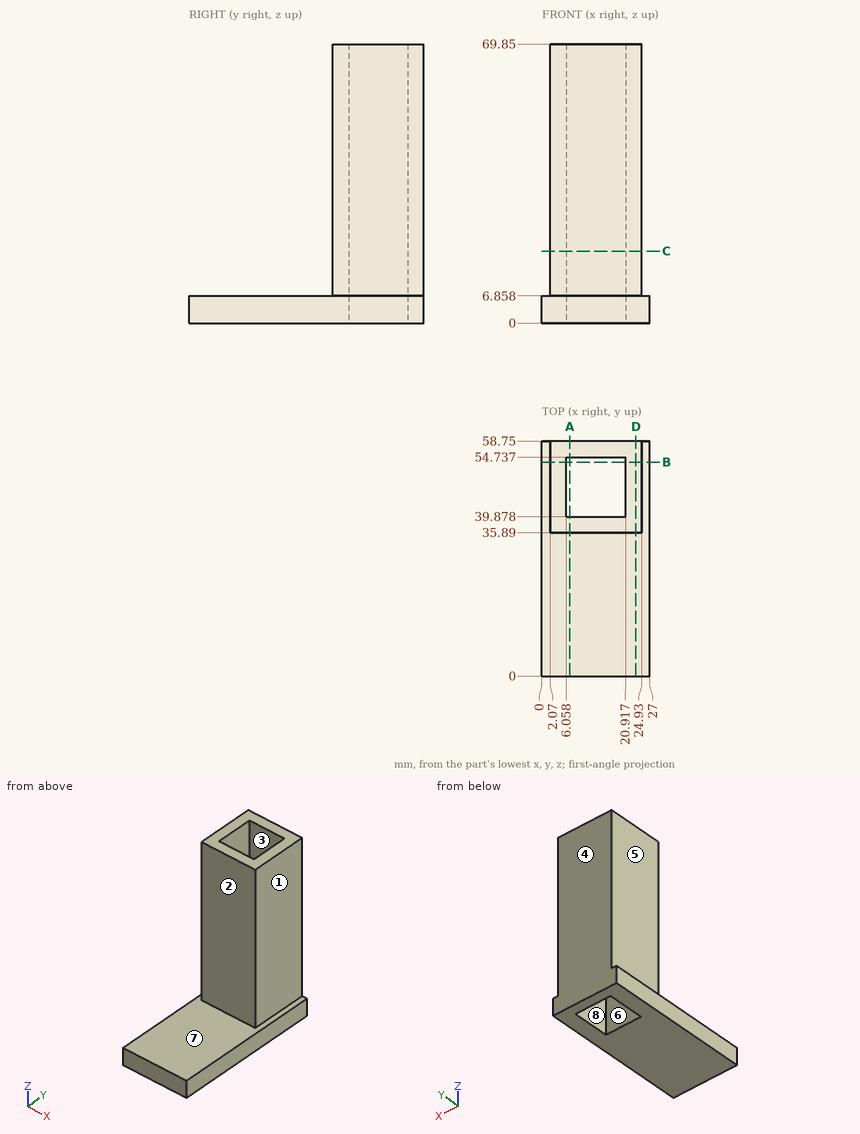
Study the drawing (mm; zero at the part's minimum x, y, z) and answer. A direction names the side the tool comes from. Give positions to 0.01 mm unless a question says otherwise; leave off trailing zeros. Write each loop counter-clockwise with the first axis right and the second up, starting at its lowest first coordinate (ties: lowest second). Pieces come first, ordered by that corner, then holes. Notation, with made-up numbers: (53, 71) -> (69, 71) arc R16 ccw to (69, 89) -> close; hole circle Ø11 at (11.5, 39). An arc over 180 degrees is marked (long way). Write item = value, one per line. Start each with the question number.
1) Determine the mould class of the marked faces 5, 6, 7 and 8 for opening direction X: +X half, -X half, draft (parallel to the pull), parting line (faces both ways), or undercut.
2) The part is cut by section D-D, the plane x = 23.5. Determine the outline of the cut face in (y, z).
3) The part is cut by section C-C, the plane z = 18. Determine the outline of the cut face in (x, y).
4) Which of the six approach directions +Z, -Z, +X, -X, +Y, -Y give full straight-line access (tool end or side, diameter ignored) to the marked faces 1, 2, 3 and 4?
5) The part is cut by section A-A, the plane x = 7. Determine the outline of the cut face in (y, z), and give its area (3 significant figures).
6) Each of these flat-tipped pins is pushed along its axis until it touches: pin 1 (1 mm diameter, centred on x = 18, z = 21.5, fed in from -Y); pin 2 (11.5 mm diameter, centred on y = 52.5, z = 29, fed in from -X); pin 3 (1.5 mm diameter, centred on x = 22, y = 27, fed in from +Z). Where does it stop, or does it pass through?
7) The part is cut by section B-B, the plane y = 53.5. Determine the outline of the cut face in (x, z), and give its area (3 significant figures).
8) Straight lines are drawn through the part: line 1 along Y through (x, z) = (17, 49); line 2 along Y through (x, z) = (16.5, 4); line 3 along X through (y, z) = (49, 42). For each, find the intervals that lie inside material, in ascending order.
Solutions:
q1.face_5 = -X half
q1.face_6 = undercut
q1.face_7 = draft
q1.face_8 = undercut
q2.outline = (0, 0) -> (58.75, 0) -> (58.75, 69.85) -> (35.89, 69.85) -> (35.89, 6.86) -> (0, 6.86) -> close
q3.outline = (2.07, 35.89) -> (24.93, 35.89) -> (24.93, 58.75) -> (2.07, 58.75) -> close; hole (6.06, 39.88) -> (20.92, 39.88) -> (20.92, 54.74) -> (6.06, 54.74) -> close
q4.face_1 = +Z, +X, +Y, -Y
q4.face_2 = +Z, +X, -X, -Y
q4.face_3 = +Z, -Z
q4.face_4 = +Z, -Z, +X, -X, +Y
q5.outline = (0, 0) -> (39.88, 0) -> (39.88, 69.85) -> (35.89, 69.85) -> (35.89, 6.86) -> (0, 6.86) -> close; (54.74, 0) -> (58.75, 0) -> (58.75, 69.85) -> (54.74, 69.85) -> close
q5.area = 805 mm²
q6.pin_1 = 35.89
q6.pin_2 = 2.07
q6.pin_3 = 6.86
q7.outline = (0, 0) -> (6.06, 0) -> (6.06, 69.85) -> (2.07, 69.85) -> (2.07, 6.86) -> (0, 6.86) -> close; (20.92, 0) -> (27, 0) -> (27, 6.86) -> (24.93, 6.86) -> (24.93, 69.85) -> (20.92, 69.85) -> close
q7.area = 587 mm²
q8.line_1 = 35.89 to 39.88, 54.74 to 58.75
q8.line_2 = 0 to 39.88, 54.74 to 58.75
q8.line_3 = 2.07 to 6.06, 20.92 to 24.93
